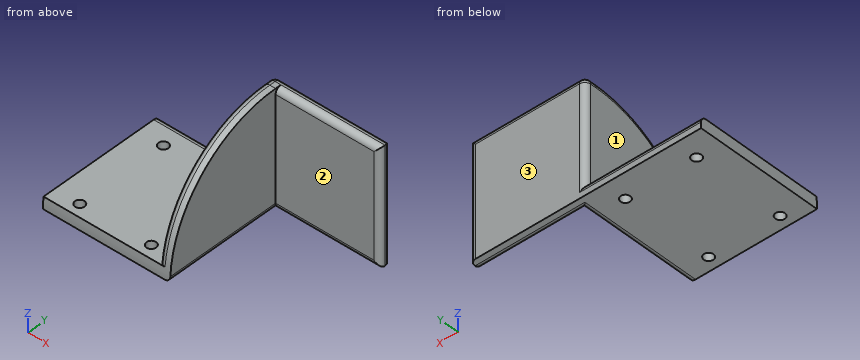
from build123d import *

# Parameters (mm, degrees)
SKETCH_1_W          = 60
SKETCH_1_H          = 60
EXTRUDE_312_DEPTH   = 6
SKETCH_2_W          = 6
SKETCH_2_H          = 60
EXTRUDE_2_DEPTH     = 60
SKETCH_3_W          = 6
SKETCH_3_H          = 66
EXTRUDE_708_DEPTH   = 60
FILLET_1_R          = 60
SKETCH_4_R          = 2.5
CUT_EXTRUDE_1_DEPTH = 6
FILLET_2_R          = 3
FILLET_3_R          = 3
FILLET_4_R          = 3
FILLET_7_R          = 3


with BuildPart() as part:
    # Эскиз1 → Extrude 312 (new body)
    with BuildSketch(Plane(origin=(0, 0, 0), x_dir=(1, 0, 0), z_dir=(0, 1, 0))):
        Rectangle(SKETCH_1_W, SKETCH_1_H)
    extrude(amount=EXTRUDE_312_DEPTH)

    # Эскиз2 → Бобышка-Вытянуть2 (add)
    with BuildSketch(Plane.XZ):
        with Locations((-27, 0)):
            Rectangle(SKETCH_2_W, SKETCH_2_H)
    extrude(amount=EXTRUDE_2_DEPTH)

    # Эскиз3 → Extrude 708 (add)
    with BuildSketch(Plane.ZY.offset(30)):
        with Locations((-27, -27)):
            Rectangle(SKETCH_3_W, SKETCH_3_H)
    extrude(amount=EXTRUDE_708_DEPTH)

    # Скругление1
    fillet_1_edges = [part.edges().sort_by_distance(p)[0] for p in [
        (-27, -60, 30),
    ]]
    fillet(fillet_1_edges, radius=FILLET_1_R - 0.0001)  # a hair under: the kernel refuses the full size

    # Эскиз4 → Вырез-Вытянуть1 (cut)
    with BuildSketch(Plane.XY.offset(-24)):
        with Locations((-76.761220605, -5.987815157)):
            Circle(SKETCH_4_R)
        with Locations((-39.838074985, -5.987815157)):
            Circle(SKETCH_4_R)
        with Locations((-76.761220605, -53.599239773)):
            Circle(SKETCH_4_R)
        with Locations((-39.838074985, -53.356324341)):
            Circle(SKETCH_4_R)
    extrude(amount=-CUT_EXTRUDE_1_DEPTH, mode=Mode.SUBTRACT)

    # Скругление2
    fillet_2_edges = [part.edges().sort_by_distance(p)[0] for p in [
        (-60, 6, -24),
    ]]
    fillet(fillet_2_edges, radius=FILLET_2_R)

    # Скругление3
    fillet_3_edges = [part.edges().sort_by_distance(p)[0] for p in [
        (3, 0, 30),
        (-24, -30, -30),
        (3, 0, -30),
        (30, 0, 0),
    ]]
    fillet(fillet_3_edges, radius=FILLET_3_R)

    # Скругление4
    fillet_4_edges = [part.edges().sort_by_distance(p)[0] for p in [
        (-30, 6, 1.5),
    ]]
    fillet(fillet_4_edges, radius=FILLET_4_R)

    # Скругление7
    fillet_7_edges = [part.edges().sort_by_distance(p)[0] for p in [
        (-30, -40.249290054, 14.497186422),
        (-30, 1.49995, 30),
        (-29.121320344, 5.121320344, 30),
        (30, 6, 0),
        (1.5, 6, 30),
    ]]
    fillet(fillet_7_edges, radius=FILLET_7_R - 0.0001)  # a hair under: the kernel refuses the full size


solid = part.part
Source: CAD feature listing. Evaluate the final solid. Frame: model axes, mm. Face numbers are marked on the shaded views. A direction names the side the tool comes from. Coordinates: 2 decimals unless noted, no trailing zeros. Answer in a Markdown table with one row per item. Add a question column.
Q1. Ray query, line 1 along X through (y, z) = (-34, 2.5); line 2 along Y through (x, z) = (-20, -13). Return the intervals inside material, ascending.
Q2. Contact query for flat-ended pins moving along their axis: pin 1 Ø5 at (x, z) = (-28.5, -2.5) entering from -Y; pin 2 Ø3 at (y, z) = (-33.5, -14) entering from +X; pin 3 Ø12 at (y, z) = (-17.5, 22) entering from -X. Output: stop coordinate, or through.
Q3. Section B-B on x = -40. Give the number of separate pieces and of enclosed holes in the cut face, and give its area (3 significant figures).
Q4. Reachability of the marked faces 1, 2 and 3 from +Z, -Z, +X, -X, +Y, -Y: full face, straight path, thin tool, end or side. Return the list, or none.
Computed values:
| question | item | result |
|---|---|---|
| 1 | line 1 | x = -30 to -24 |
| 1 | line 2 | y = 0 to 6 |
| 2 | pin 1 | stops at y = -54.4 |
| 2 | pin 2 | stops at x = -24 |
| 2 | pin 3 | stops at x = -30 |
| 3 | separate pieces | 3 |
| 3 | enclosed holes | 0 |
| 3 | area | 334 mm^2 |
| 4 | face 1 | +Z, -X, +Y, -Y |
| 4 | face 2 | +Z, -Z, +X, -Y |
| 4 | face 3 | +Z, -Z, +X, -X, +Y |
